For this review, use the dimensioned drawing (mm, ordinates from the lowest corner) and the shaded views. A direction names the side the tool comes from. Round coordinates to 2 decimals unless told otherwise and drop trailing zeros. Loops run counter-clockwise (first coordinate to the right, second up) from the corner with the lowest first, then second, coordinate; pieces in that order, holes last. Notation, with made-up numbers: (57, 82.5) -> (89, 82.5) arc R32 cw to (89, 115.5) -> close; hole circle Ø2 at (26.5, 43.25). An arc over 180 degrees is marked (long way). Use one line per item in the form item = value. Start each with the question number.
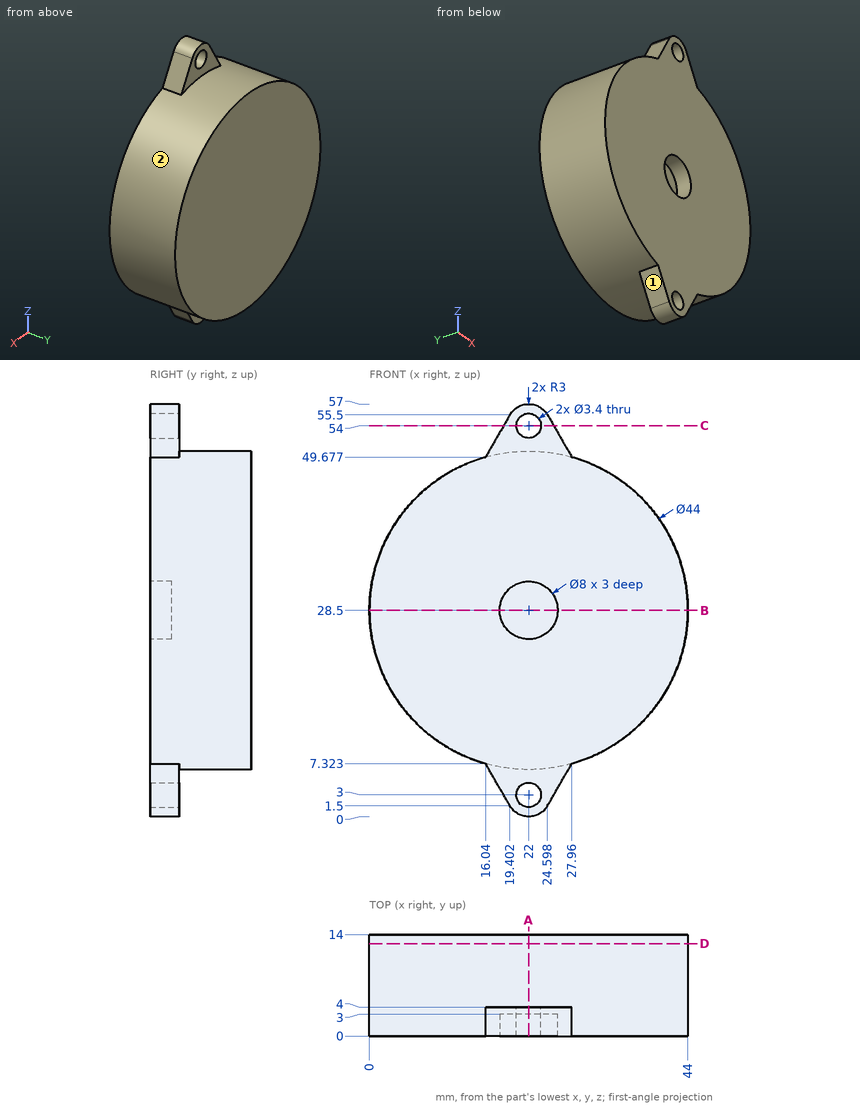
Item 1: Wall thickness on line 1 (X direction, y = 2, z = 28.5); line 2 (Y direction, x = 20, z = 28.5); line 3 (Z direction, x = 23.5, y = 2.25) (1 decimal): over which ranges is each line inside the solid? List them lowest first.
Item 2: Take a section at B-B on z = 28.5. Give the boundary of the cut face in (x, y).
Item 3: Machinability: for the marked faces 1 and 2, which of the approach directions +Z, -Z, +X, -X, +Y, -Y give a long, thin tool a straight path to every point of the face, cutting with its end or side? Answer none if there is none.
Item 4: Take a section at D-D on y = 12.75. Give the boundary of the cut face in (x, z).
Item 5: For P1, Ø5, axis at x = 32.5, y = 4, coming from the +Z side; P2, Ø1.5, axis at x = 16, y = 4.5, coming from the +Z side (1 decimal); P3, Ø3, axis at x = 22, z = 3, coming from the -Y side; P4, Ø6, axis at x = 15, y = 5.5, coming from the -Z side (1 decimal), all flat-tipped, find the tip position at first contact; note any pin that passes through.
Item 6: Take a section at C-C on z = 54. Give the boundary of the cut face in (x, y), plus the area to 3 significant figures.
Item 7: Take a section at A-A on x = 22. Give the boundary of the cut face in (y, z), plus the area to 3 significant figures.
Results:
q1.line_1 = 0 to 18, 26 to 44
q1.line_2 = 3 to 14
q1.line_3 = 0.4 to 2.2, 3.8 to 24.8, 32.2 to 53.2, 54.8 to 56.6
q2.outline = (0, 0) -> (18, 0) -> (18, 3) -> (26, 3) -> (26, 0) -> (44, 0) -> (44, 14) -> (0, 14) -> close
q3.face_1 = -Z, -X, +Y, -Y
q3.face_2 = +Y
q4.outline = circle Ø44 at (22, 28.5)
q5.P1 = 48.99
q5.P2 = 50.6
q5.P3 = through
q5.P4 = 4.6
q6.outline = (18.54, 0) -> (20.3, 0) -> (20.3, 4) -> (18.54, 4) -> close; (23.7, 0) -> (25.46, 0) -> (25.46, 4) -> (23.7, 4) -> close
q6.area = 14.1 mm2
q7.outline = (0, 0) -> (4, 0) -> (4, 1.3) -> (0, 1.3) -> close; (0, 4.7) -> (4, 4.7) -> (4, 6.5) -> (14, 6.5) -> (14, 50.5) -> (4, 50.5) -> (4, 52.3) -> (0, 52.3) -> (0, 32.5) -> (3, 32.5) -> (3, 24.5) -> (0, 24.5) -> close; (0, 55.7) -> (4, 55.7) -> (4, 57) -> (0, 57) -> close
q7.area = 617 mm2
